Can you work these out from the model? Positions are in its coordinate system, mm. A direction names the side the tool comes from. Give positions to 0.01 mm unless a question says otherwise; leave off trailing zeros. Loops run counter-clockwise (first coordinate to the right, second up) from the corner with the lowest first, then second, coordinate; pieces in that order, holes last. Notation, with made-up numbers: (18, -2) - (70, -2) arc R19 cw to (70, 17) - close; hole circle Ø2 at (62, -15). An arc over 180 degrees is marked (long way). Answer as a JSON object with one key per item and string values. Group by question number.
Item 1: Suppose I cut it at B-B on x = 69.5. Write out the boundary of the cut face in (y, z).
Item 2: Suppose I cut it at A-A on x = 33.5. Write out the boundary of the cut face in (y, z).
Item 3: Suppose I cut it at D-D on x = 12.5. Write out the boundary of the cut face in (y, z).
Item 4: Thinking about a two-plate mould opening in Y: for faces 4 (the cylindrical face through (20.28, -1.15, -2.77)), 5 (the cylindrical face through (8, -6, 0)), 6 (the conical face through (46.49, -0.51, -0.11)), 7 (the flat face through (65, -2, -6)), which applies, pulls with the +Y half, pulls with the -Y half, needs draft (parallel to the pull), parting line crosses it, or undercut?
Item 5: Suppose I cut it at C-C on z = -6.75. Write out the boundary of the cut face in (x, y), and give its area (3 significant figures).
Item 6: Please list where these lines run through material, in increasing order: L1, parallel to X at y = 0, z = -4.5; L2, parallel to X at y = 7, z = -2.25; L3, parallel to Y at x = 32, z = -0.25.
Item 7: Will these pins go through, and if not, where does the flat tip stop? pin 1 (5 mm diameter, centred on x = 33.5, y = 5, fed in from -Z); pin 2 (3 mm diameter, centred on y = 1.5, z = -6.5, fed in from -X); pin 3 (3.5 mm diameter, centred on y = 0, z = 0, fed in from -X); pin 4 (8 mm diameter, centred on x = 40, y = 0, fed in from -Z).
Item 8: Which directions (+Z, -Z, +X, -X, +Y, -Y) give clear straight access to the entire face, cutting with the end or side of a thin tool? Please do faces 1 (the flat face through (0, 3.3, 0.1)), 2 (the cylindrical face through (43.09, -2.93, 0.65)), 3 (the cylindrical face through (72, -6, 0)).
from build123d import *

# Parameters (mm, degrees)
SKETCH2_R                    = 3
CUT_EXTRUDE1_DEPTH           = 10
CUT_EXTRUDE1_DEPTH_BACK      = 10
CHAMFER1_SIZE                = 1
F_6_0_6_DIAMETER_HOLE1_D     = 6
F_6_0_6_DIAMETER_HOLE1_DEPTH = 45
F_6_0_6_DIAMETER_HOLE1_TIP   = 1.802581857


with BuildPart() as part:
    # Sketch1 → Revolve1 (revolve)
    with BuildSketch(Plane.XY):
        Polygon((0, 0), (80, 0), (80, 6), (65, 6), (65, 9), (15, 9), (15, 6), (0, 6), align=None)
    revolve(axis=Axis((0, 0, 0), (1, 0, 0)))

    # Sketch2 → Cut-Extrude1 (cut, two sides)
    with BuildSketch(Plane.XY) as cut_extrude1_sk:
        with Locations((40, 0)):
            Circle(SKETCH2_R)
    extrude(amount=CUT_EXTRUDE1_DEPTH, mode=Mode.SUBTRACT)
    extrude(cut_extrude1_sk.sketch, amount=-CUT_EXTRUDE1_DEPTH_BACK, mode=Mode.SUBTRACT)

    # Chamfer1
    chamfer1_edges = [part.edges().sort_by_distance(p)[0] for p in [
        (0, -6, 0),
        (80, -6, 0),
    ]]
    chamfer(chamfer1_edges, length=CHAMFER1_SIZE)

    # Ø6.0 (6) Diameter Hole1
    with Locations(Plane.ZY):
        with Locations((0, 0)):
            Hole(F_6_0_6_DIAMETER_HOLE1_D / 2, depth=F_6_0_6_DIAMETER_HOLE1_DEPTH)
            with Locations((0, 0, -(F_6_0_6_DIAMETER_HOLE1_DEPTH + F_6_0_6_DIAMETER_HOLE1_TIP / 2))):  # 118° drill point
                Cone(0, F_6_0_6_DIAMETER_HOLE1_D / 2, F_6_0_6_DIAMETER_HOLE1_TIP, mode=Mode.SUBTRACT)


solid = part.part
Worked out:
{
 "1": {"outline": "circle Ø12 at (0, 0)"},
 "2": {"outline": "circle Ø18 at (0, 0); hole circle Ø6 at (0, 0)"},
 "3": {"outline": "circle Ø12 at (0, 0); hole circle Ø6 at (0, 0)"},
 "4": {"face 4": "undercut", "face 5": "parting line crosses it", "face 6": "undercut", "face 7": "needs draft"},
 "5": {"outline": "(15, -5.95) - (65, -5.95) - (65, 5.95) - (15, 5.95) - close; hole circle Ø6 at (40, 0)", "area": "567 mm2"},
 "6": {"L1": "x = 0 to 37, 43 to 80", "L2": "x = 15 to 65", "L3": "y = -9 to -2.99, 2.99 to 9"},
 "7": {"pin 1": "stops at z = -8.65", "pin 2": "stops at x = 0.17", "pin 3": "stops at x = 45.75", "pin 4": "stops at z = -9"},
 "8": {"face 1": "+Z, -Z, -X, +Y, -Y", "face 2": "-X", "face 3": "+X"}
}
